Autodesk Inventor part; units mm, degrees
ref_plane "YZ Plane" through (0, 0, 0) normal (1, 0, 0) x (0, 1, 0)
ref_plane "XZ Plane" through (0, 0, 0) normal (0, 1, 0) x (-1, 0, 0)
ref_plane "XY Plane" through (0, 0, 0) normal (0, 0, 1) x (1, 0, 0)
sketch "Sketch1" plane through (0, 0, 0) normal (0, 1, 0) x (-1, 0, 0)
  line L0 (0, 0) -> (50.8, 0)
  line L1 (50.8, 0) -> (50.8, -736.6)
  line L2 (50.8, -736.6) -> (0, -736.6)
  line L3 (0, -736.6) -> (0, 0)
  dimension "d0" = 50.8
  dimension "d1" = 736.6
extrude "Extrusion1" add sketch "Sketch1" along normal blind 6.35
sketch "Sketch2" plane through (0, 6.35, 0) normal (0, 1, 0) x (1, 0, 0)
  line L0 (-50.8, 0) -> (-44.45, 0)
  line L1 (-50.8, 0) -> (0, 0)
  line L2 (-44.45, 0) -> (-44.45, 736.6)
  line L3 (0, 736.6) -> (-50.8, 736.6)
  line L4 (-44.45, 736.6) -> (-50.8, 736.6)
  line L5 (-50.8, 736.6) -> (-50.8, 0)
  line L6 (-50.8, 0) -> (-44.45, 0)
  dimension "d4" = 6.35
  dimension "d5" = 736.6
  dimension "d6" = 736.6
extrude "Extrusion2" add sketch "Sketch2" along normal blind 44.45
fillet "Fillet1" radius 6.35 1 edges at (-44.45, 6.35, -368.3)
fillet "Fillet2" radius 6.35 1 edges at (0, 6.35, -368.3)
fillet "Fillet3" radius 6.35 1 edges at (-44.45, 50.8, -368.3)
hole "Hole1" at (-44.45, 25.4, -247.65) direction (-1, 0, 0) diameter 9.525 end through all
pattern_linear "Rectangular Pattern1" count 3 spacing 152.4 along (0, 0, -1) of "Hole1"
hole "Hole2" at (-44.45, 25.4, -671.6014) direction (-1, 0, 0) diameter 15.24 end through all
properties part number "2x2 quarter in angle aluminum"
The model under review builds one solid part; all positions refer to its coordinate system, in mm. A direction names the side the tool comes from. Round coordinates to 2 decimals unless told otherwise and drop trailing zeros.
(1) Wall thickness on L1, parallel to Z at x = -49.25, y = 25.4; L2, parallel to Y at x = -18.5, z = -312.5; L3, parallel to Y at x = -48.75, z = -400.05: over which ranges is each line inside the solid? List them lowest first.
(2) Insertion check: pin 1 (10 mm diameter, centred on y = 34, z = -169.5, fed in from +X); pin 2 (5.5 mm diameter, centred on y = 25.4, z = -400.05, fed in from +X); pin 3 (9.5 mm diameter, centred on x = -14.5, z = -256.5, fed in from +Y). Each pin has a flat end and moves straight along its axis. Give the tip position at first contact, or say it passes through.
(3) Mouldability with a two-part tool opening along Z and no side actions: class faces 3 (the flat face through (-40, 6, 0)), 4 (the flat face through (-25, 0, -363)), 5 (the cylindrical face through (-47.67, 32.16, -675.12)) as +Z half, -Z half, draft (parallel to the pull), parting line (faces both ways), or undercut.
(4) Machinability: for faces 1 (the flat face through (-44.45, 28, -363)), 2 (the flat face through (-44.3, 10.2, -736.6)), which of the approach directions +Z, -Z, +X, -X, +Y, -Y give a long, thin tool a straight path to every point of the face, cutting with its end or side? Answer none if there is none.
Findings below:
1. L1: z = -736.6 to -679.22, -663.98 to -557.21, -547.69 to -404.81, -395.29 to -252.41, -242.89 to 0
1. L2: y = 0 to 6.35
1. L3: y = 0 to 20.64, 30.16 to 50.46
2. pin 1: stops at x = -44.45
2. pin 2: passes through
2. pin 3: stops at y = 6.35
3. face 3: +Z half
3. face 4: draft
3. face 5: undercut
4. face 1: +Z, -Z, +X, +Y
4. face 2: -Z, +X, -X, +Y, -Y
